Read the model definition and answer for the solid it produces. Units are mm, in the model's axes. A direction names the side the tool comes from. Coordinates: 2 decimals unless noted, no trailing zeros. Loops run counter-clockwise (first coordinate to the right, second up) from the corner with the lowest first, then second, coordinate; pieces in that order, holes last. Notation, with made-up numbers: (16.5, 6) -> (38.5, 6) arc R17 cw to (38.5, 30) -> close; hole circle Ø3 at (50.5, 13.25). An arc over 180 degrees is marked (long way). Answer as a JSON object with one key per item and string values. Group by question number.
1) Which of the six approach directions +Z, -Z, +X, -X, +Y, -Y give full straight-line access (tool end or side, diameter ignored) to faces 1 (the face through (-13.983, 1.479, -20.873)), 2 (the face through (0, 5, 22)), 3 (the face through (0, 5, -22)), 4 (the face through (10, 17, -17)), 5 (the face through (-28.75, 10.35, -0.07))?
2) Section A-A, the plane x = 0 is taken. Give the vertices of the cut face in (y, z), plus the area to 3 significant figures.
3) Section B-B, the plane z = 0 is taken. Count the separate pieces of the cut face and the enclosed holes in it, plus the area to 3 significant figures.
4) Section D-D, the plane y = 16.25 is taken. Give the vertices of the cut face in (x, z) (3 decimals).
5) Consider probe 1 along Z at (x, y) = (-13, 9.5); probe 2 along Z at (x, y) = (23.5, 5.75); probe 3 along Z at (x, y) = (13.5, 16.5). Determine where each line is inside the solid, lowest interval first. Write a range as [from, to].
6) Flat-ended cylindrical pins translate along their axes: P1, Ø6, axis at x = -20, y = 5, coming from the -Z side; P2, Ø2, axis at y = 8, z = 22.5, coming from the -X side; P3, Ø4.5, axis at x = 27.25, z = 0, coming from the -Y side; P4, Ø1.8, axis at x = -13.62, z = 23.6, coming from the -Y side. Find the tip coordinate at first contact, or state that the pin passes through.
from build123d import *

# Parameters (mm, degrees)
SKETCH_1_R               = 32
SKETCH_1_R_2             = 2.5
SKETCH_1_R_3             = 1.5
EXTRUDE_1_DEPTH          = 20
SKETCH_2_R               = 2.75
CUT_EXTRUDE_1_DEPTH      = 2.1
SKETCH_3_R               = 2.5
CUT_EXTRUDE_2_DEPTH      = 3
SKETCH_4_R               = 2
CUT_EXTRUDE_3_DEPTH      = 10
PATTERN_CIRCULAR_1_COUNT = 6
SKETCH_5_R               = 15
CUT_EXTRUDE_4_DEPTH      = 21.0000001
SKETCH_6_R               = 2.75
SKETCH_6_R_2             = 1.5
CUT_EXTRUDE_5_DEPTH      = 3


with BuildPart() as part:
    # 草图1 → 凸台-拉伸1 (new body)
    with BuildSketch(Plane(origin=(0, 0, 0), x_dir=(1, 0, 0), z_dir=(0, 1, 0))):
        Circle(SKETCH_1_R)
        with Locations((-23.599192253, -13.625)):
            Circle(SKETCH_1_R_2, mode=Mode.SUBTRACT)
        with Locations((-13.625, -23.599192253)):
            Circle(SKETCH_1_R_3, mode=Mode.SUBTRACT)
        with Locations((0, -27.25)):
            Circle(SKETCH_1_R_2, mode=Mode.SUBTRACT)
        with Locations((13.625, -23.599192253)):
            Circle(SKETCH_1_R_3, mode=Mode.SUBTRACT)
        with Locations((23.599192253, -13.625)):
            Circle(SKETCH_1_R_2, mode=Mode.SUBTRACT)
        with Locations((27.25, 0)):
            Circle(SKETCH_1_R_3, mode=Mode.SUBTRACT)
        with Locations((23.599192253, 13.625)):
            Circle(SKETCH_1_R_2, mode=Mode.SUBTRACT)
        with Locations((13.625, 23.599192253)):
            Circle(SKETCH_1_R_3, mode=Mode.SUBTRACT)
        with Locations((0, 27.25)):
            Circle(SKETCH_1_R_2, mode=Mode.SUBTRACT)
        with Locations((-13.625, 23.599192253)):
            Circle(SKETCH_1_R_3, mode=Mode.SUBTRACT)
        with Locations((-23.599192253, 13.625)):
            Circle(SKETCH_1_R_2, mode=Mode.SUBTRACT)
        with Locations((-27.25, 0)):
            Circle(SKETCH_1_R_3, mode=Mode.SUBTRACT)
        with Locations((-23.599192253, -13.625)):
            Circle(SKETCH_1_R_2)
        with Locations((-23.599192253, 13.625)):
            Circle(SKETCH_1_R_2)
        with Locations((23.599192253, 13.625)):
            Circle(SKETCH_1_R_2)
        with Locations((0, 27.25)):
            Circle(SKETCH_1_R_2)
        with Locations((0, -27.25)):
            Circle(SKETCH_1_R_2)
        with Locations((23.599192253, -13.625)):
            Circle(SKETCH_1_R_2)
    extrude(amount=EXTRUDE_1_DEPTH)

    # 草图2 → 切除-拉伸1 (cut)
    with BuildSketch(Plane(origin=(0, 20, 0), x_dir=(1, 0, 0), z_dir=(0, 1, 0))):
        with Locations((-27.25, 0)):
            Circle(SKETCH_2_R)
        with Locations((13.625, 23.599192253)):
            Circle(SKETCH_2_R)
        with Locations((13.625, -23.599192253)):
            Circle(SKETCH_2_R)
    extrude(amount=-CUT_EXTRUDE_1_DEPTH, mode=Mode.SUBTRACT)

    # 草图3 → 切除-拉伸2 (cut)
    with BuildSketch(Plane(origin=(0, 20, 0), x_dir=(1, 0, 0), z_dir=(0, 1, 0))):
        with Locations((-19.55, 0)):
            Circle(SKETCH_3_R)
        with Locations((9.775, 16.930796644)):
            Circle(SKETCH_3_R)
        with Locations((9.775, -16.930796644)):
            Circle(SKETCH_3_R)
    extrude(amount=-CUT_EXTRUDE_2_DEPTH, mode=Mode.SUBTRACT)

    # 草图4 → 切除-拉伸3 (cut)
    with BuildSketch(Plane.XY.offset(32)):
        with Locations((0, 5)):
            Circle(SKETCH_4_R)
    cut_extrude_3 = extrude(amount=-CUT_EXTRUDE_3_DEPTH, mode=Mode.SUBTRACT)

    # 阵列(圆周)1: 切除-拉伸3 ×6 about axis
    pattern_circular_1_axis = Axis((0, 0, 0), (0, 1, 0))
    for i in range(1, PATTERN_CIRCULAR_1_COUNT):
        add(cut_extrude_3.rotate(pattern_circular_1_axis, i * 360 / PATTERN_CIRCULAR_1_COUNT), mode=Mode.SUBTRACT)

    # 草图5 → 切除-拉伸4 (cut, through all)
    with BuildSketch(Plane(origin=(0, 20, 0), x_dir=(1, 0, 0), z_dir=(0, 1, 0))):
        Circle(SKETCH_5_R)
    extrude(amount=-CUT_EXTRUDE_4_DEPTH, mode=Mode.SUBTRACT)

    # 草图6 → 切除-拉伸5 (cut)
    with BuildSketch(Plane.XZ):
        with Locations((13.625, -23.599192253)):
            Circle(SKETCH_6_R)
        with Locations((13.625, -23.599192253)):
            Circle(SKETCH_6_R_2, mode=Mode.SUBTRACT)
        with Locations((27.25, 0)):
            Circle(SKETCH_6_R)
        with Locations((27.25, 0)):
            Circle(SKETCH_6_R_2, mode=Mode.SUBTRACT)
        with Locations((13.625, 23.599192253)):
            Circle(SKETCH_6_R)
        with Locations((13.625, 23.599192253)):
            Circle(SKETCH_6_R_2, mode=Mode.SUBTRACT)
        with Locations((-13.625, 23.599192253)):
            Circle(SKETCH_6_R)
        with Locations((-13.625, 23.599192253)):
            Circle(SKETCH_6_R_2, mode=Mode.SUBTRACT)
        with Locations((-27.25, 0)):
            Circle(SKETCH_6_R)
        with Locations((-27.25, 0)):
            Circle(SKETCH_6_R_2, mode=Mode.SUBTRACT)
        with Locations((-13.625, -23.599192253)):
            Circle(SKETCH_6_R)
        with Locations((-13.625, -23.599192253)):
            Circle(SKETCH_6_R_2, mode=Mode.SUBTRACT)
    extrude(amount=-CUT_EXTRUDE_5_DEPTH, mode=Mode.SUBTRACT)


solid = part.part
Determined:
{
 "1": {"face 1": "-Y", "face 2": "+Z", "face 3": "-Z", "face 4": "+Y", "face 5": "+Y, -Y"},
 "2": {"outline": "(0, -32) -> (3, -32) -> (3, -22) -> (7, -22) -> (7, -32) -> (20, -32) -> (20, -15) -> (0, -15) -> close; (0, 15) -> (20, 15) -> (20, 32) -> (7, 32) -> (7, 22) -> (3, 22) -> (3, 32) -> (0, 32) -> close", "area": "600 mm²"},
 "3": {"separate pieces": "4", "enclosed holes": "0", "area": "525 mm²"},
 "4": {"outline": "circle Ø64 at (0, 0); hole circle Ø3 at (-27.25, 0); hole circle Ø3 at (-13.625, -23.599); hole circle Ø3 at (-13.625, 23.599); hole circle Ø30 at (0, 0); hole circle Ø3 at (13.625, -23.599); hole circle Ø3 at (13.625, 23.599); hole circle Ø3 at (27.25, 0)"},
 "5": {"probe 1": "[-29.24, -24.96], [-22.24, -7.48], [7.48, 22.24], [24.96, 29.24]", "probe 2": "[-21.72, -15.71], [-11.43, 11.43], [15.71, 21.72]", "probe 3": "[-29.01, -25.09], [-22.1, -6.54], [6.54, 22.1], [25.09, 29.01]"},
 "6": {"P1": "z = -27.11", "P2": "x = -23.7", "P3": "y = 3", "P4": "through"}
}
